Source: CAD feature listing. Evaluate the final solid. Frame: model axes, mm. A direction names the side the tool comes from. Give positions to 0.01 mm unless a question says otherwise; leave off trailing zeros. Write each loop counter-clockwise with the first axis right and the second up, starting at its lowest first coordinate (ties: lowest second). Pieces come first, ordered by that corner, then holes. Notation, with made-up numbers: (73, 7.25) - (121, 7.25) arc R9 cw to (121, 22.25) - close; hole circle Ø8 at (-10, 56.5). An arc over 180 degrees is marked (long way). One line per question, with ' | ' between items. Start each with the question number.
(1) Section C-C, the plane x = -8. Return loops of the section in (y, z), plus the area to 3 significant figures.
(2) Ray query, line 1 (Y direction, x = -8, z = 2.75); line 2 (Y direction, x = 12, z = 1); line 3 (Y direction, x = -9.5, z = 3.25). Return the intervals inside material, ascending. Write a range as [from, to].
(3) Section D-D, the plane z = 7. Return loops of the section in (x, y), plus the area to 3 significant figures.
(4) Section A-A, the plane x = -0.25. Return loops of the section in (y, z), plus the area to 3 significant figures.
(5) Access query for faces 1 (the cylindrical face through (-5.8, -9.55, 4.06)), 2 (the flat face through (-7, 0, 0)). Directions: +Z, -Z, +X, -X, +Y, -Y. A direction counts if a zero-diameter tool reaches every point of the face in a straight line with its end or side. Return the directions, or none.
(6) Draft query along Y for faces 3 (the flat face through (0, -22.5, 4)), 4 (the flat face through (5, 10, 4)), 5 (the flat face through (-6.228, 0, 4)), 6 (the flat face through (15, -16, 4)). Return one class per face: +Y half, -Y half, draft (parallel to the pull), parting line (faces both ways), or undercut.
(7) Section B-B, the plane y = 17.5. Return loops of the section in (x, z), plus the area to 3 significant figures.
(8) Pin query (flat end, axial travel): pin 1 (2.5 mm diameter, centred on y = 0.5, z = 5.5, fed in from +X). Return the tip coordinate at first contact, or that it passes through.
Autodesk Inventor part; units mm, degrees
ref_plane "YZ Plane" through (0, 0, 0) normal (1, 0, 0) x (0, 1, 0)
ref_plane "XZ Plane" through (0, 0, 0) normal (0, 1, 0) x (-1, 0, 0)
ref_plane "XY Plane" through (0, 0, 0) normal (0, 0, 1) x (1, 0, 0)
sketch "Sketch1" plane through (0, 0, 0) normal (0, 0, 1) x (1, 0, 0)
  line L0 (-15, 22.5) -> (15, 22.5)
  line L1 (15, 22.5) -> (15, -22.5)
  line L2 (15, -22.5) -> (-15, -22.5)
  line L3 (-15, -22.5) -> (-15, 22.5)
  point P0 (0, 0)
  point P1 (0, 22.5)
  point P2 (-15, 0)
  dimension "d0" = 30
  dimension "d1" = 45
extrude "Extrusion1" add sketch "Sketch1" along normal blind 8
sketch "Sketch3" plane through (0, 0, 0) normal (0, 0, -1) x (-1, 0, 0)
  arc A0 (6.2282, -0.4043) -> (6.2368, 0) centre (-3.25, 0) ccw
  line L0 (6.2282, -10) -> (-15, -10)
  line L1 (-15, -10) -> (-15, 10)
  line L2 (-15, 10) -> (6.2282, 10)
  line L3 (6.2282, 10) -> (6.2282, -10)
  line L4 (15, 22.5) -> (15, -22.5)
  line L5 (-15, -22.5) -> (-15, 22.5)
  point P0 (0, 0)
  point P1 (6.2282, 0)
  point P2 (15, 0)
  dimension "d8" = 0
  dimension "d9" = 20
extrude "Extrusion3" cut sketch "Sketch3" against normal blind 10
sketch "Sketch4" plane through (0, 0, 0) normal (0, 0, -1) x (-1, 0, 0)
  line L0 (-15, -22.5) -> (-15, -10)
  line L1 (-15, 10) -> (-15, 22.5)
  circle A0 centre (8, 17.5) radius 1.75
  circle A1 centre (8, -17.5) radius 1.75
  line L2 (-15, 22.5) -> (15, 22.5)
  line L3 (15, 22.5) -> (15, -22.5)
  line L4 (15, -22.5) -> (-15, -22.5)
  point P0 (-15, -16.25)
  point P1 (-15, 16.25)
  dimension "d17" = 3.5
  dimension "d18" = 3.5
  dimension "d19" = 5
  dimension "d20" = 7
  dimension "d21" = 5
  dimension "d22" = 35
extrude "Extrusion4" cut sketch "Sketch4" against normal through all
fillet "Fillet1" radius 1.5 2 edges at (-6.2282, -10, 4) (-6.2282, 10, 4)
equation "\"d21\" = d19"
properties part number "0005-10-004 Actionare 2 seringa"
Check sheet entries:
1) outline: (-22.5, 0) - (-19.25, 0) - (-19.25, 8) - (-22.5, 8) - close; (-15.75, 0) - (15.75, 0) - (15.75, 8) - (-15.75, 8) - close; (19.25, 0) - (22.5, 0) - (22.5, 8) - (19.25, 8) - close | area: 304 mm²
2) line 1: [-22.5, -19.25], [-15.75, 15.75], [19.25, 22.5] | line 2: [-22.5, -10], [10, 22.5] | line 3: [-22.5, -18.4], [-16.6, 16.6], [18.4, 22.5]
3) outline: (-15, -22.5) - (15, -22.5) - (15, -10) - (-4.73, -10) arc R1.5 cw to (-6.23, -8.5) - (-6.23, 8.5) arc R1.5 cw to (-4.73, 10) - (15, 10) - (15, 22.5) - (-15, 22.5) - close; hole circle Ø3.5 at (-8, -17.5); hole circle Ø3.5 at (-8, 17.5) | area: 907 mm²
4) outline: (-22.5, 0) - (-10, 0) - (-10, 8) - (-22.5, 8) - close; (10, 0) - (22.5, 0) - (22.5, 8) - (10, 8) - close | area: 200 mm²
5) face 1: +Z, -Z, +X | face 2: -Z, +X, -X, +Y, -Y
6) face 3: -Y half | face 4: undercut | face 5: undercut | face 6: draft
7) outline: (-15, 0) - (-9.75, 0) - (-9.75, 8) - (-15, 8) - close; (-6.25, 0) - (15, 0) - (15, 8) - (-6.25, 8) - close | area: 212 mm²
8) pin 1: x = -6.23
